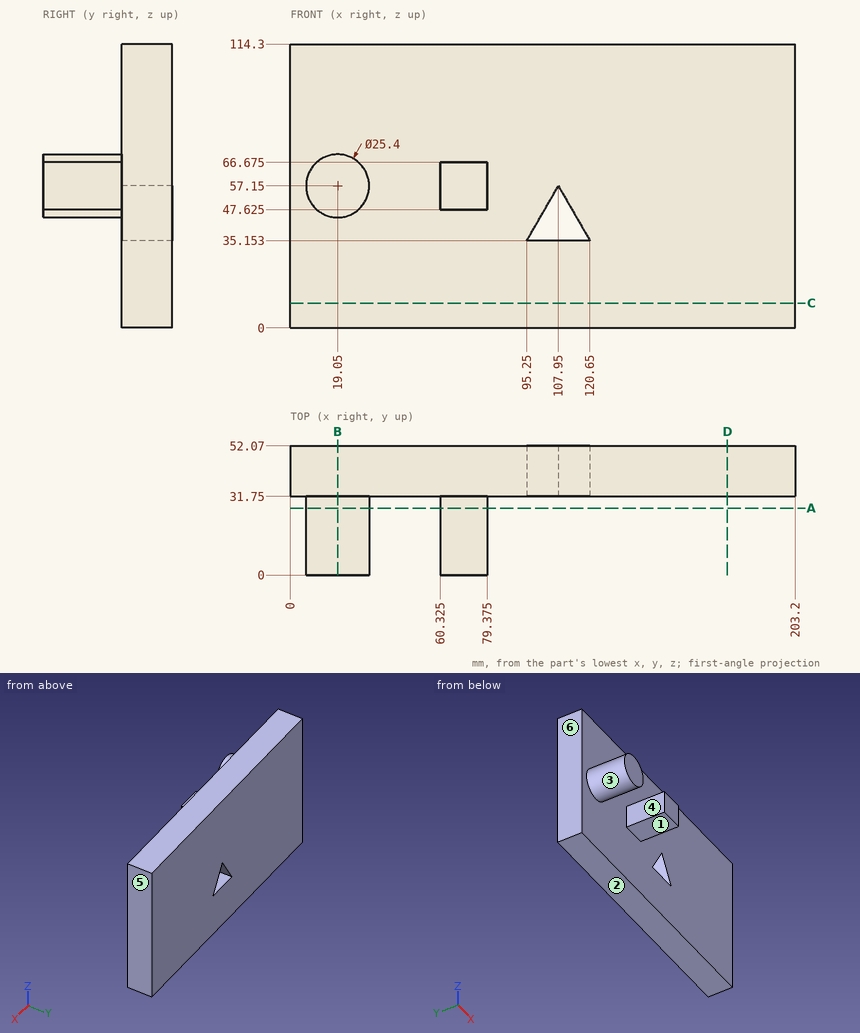
Verification items for this drawing (mm, ordinates from the low corner). A direction names the side the tool comes from. Round coordinates to 2 decimals unless told otherwise and drop trailing zeros. Order: outer loops, then holes, each group sorted by start corner. A loop starts at its lowest first (then second) coordinate and runs counter-clockwise, first axis right, second up. Notation, with made-up numbers: M 89,56 L 132,56 A7 cw 132,66 Z; hole C 19.5,3 d1. An arc over 180 degrees is marked long. Answer in a Markdown table with one row per item. Add a question column.
Item 1: Material ranges on L1, parallel to Y at x = 100, z = 35; L2, parallel to X at y = 35, z = 56.5; L3, parallel to X at y = 29, z = 51 (1 decimal), recorded low to high. Write a range as [from, to].
Item 2: Sectioned sample at B-B, the plane x = 19.05. Enter the section's corners in (y, z), plus the area to 3 significant figures.
Item 3: Sectioned sample at C-C, the plane z = 10. Enter the section's corners in (x, y).
Item 4: Sectioned sample at D-D, the plane x = 176. Enter the section's corners in (y, z).
Item 5: Sectioned sample at A-A, the plane y = 27. Enter the section's corners in (x, z) (3 decimals).
Item 6: Depth check by flat-ended pin: pin 1 Ø9.5 at (x, y) = (66, 14) entering from -Z (3 decimals); pin 2 Ø1.5 at (x, z) = (118.5, 15) entering from -Y; pin 3 Ø6 at (y, z) = (35.5, 101) entering from -X; pin 4 Ø21 at (y, z) = (17, 60) entering from +X (3 decimals). Enter the tip coordinate at first touch or a pass-through.
Item 7: Set-up check for the marked faces 1 and 2: record each of +Z, -Z, +X, -X, +Y, -Y from which the full face is reachable in a straight line by a thin tool's end or side.
Item 8: Draft check along X on the marked faces 3, 4, 5 and 6. Enter one of: released by +X, released by -X, zero draft, split by the parting line, or undercut.
Filled in:
| question | item | result |
|---|---|---|
| 1 | L1 | y = [31.75, 52.07] |
| 1 | L2 | x = [0, 107.57], [108.33, 203.2] |
| 1 | L3 | x = [7.9, 30.2], [60.3, 79.4] |
| 2 | outline | M 0,44.45 L 31.75,44.45 L 31.75,0 L 52.07,0 L 52.07,114.3 L 31.75,114.3 L 31.75,69.85 L 0,69.85 Z |
| 2 | area | 3,130 mm² |
| 3 | outline | M 0,31.75 L 203.2,31.75 L 203.2,52.07 L 0,52.07 Z |
| 4 | outline | M 31.75,0 L 52.07,0 L 52.07,114.3 L 31.75,114.3 Z |
| 5 | outline | C 19.05,57.15 d25.4; M 60.325,47.625 L 79.375,47.625 L 79.375,66.675 L 60.325,66.675 Z |
| 6 | pin 1 | stops at z = 47.625 |
| 6 | pin 2 | stops at y = 31.75 |
| 6 | pin 3 | stops at x = 0 |
| 6 | pin 4 | stops at x = 79.375 |
| 7 | face 1 | -Z, +X, -Y |
| 7 | face 2 | -Z, +X, -X, +Y, -Y |
| 8 | face 3 | undercut |
| 8 | face 4 | undercut |
| 8 | face 5 | released by +X |
| 8 | face 6 | released by -X |
